Here's the drawing with two shaded views (mm, measured from the low corner). I have some questions. A direction names the side the tool comes from. Coordinates: 2 decimals unless noted, no trailing zeros. Write each loop counter-clockwise with the first axis right and the second up, starting at its lowest first coordinate (ties: lowest second). Pieces come first, ordered by that corner, then holes.
Item 1: If we section it at D-D (x = 28): Please give me the cut outline in (y, z).
Item 2: If we section it at B-B (x = 35): Please give me the cut outline in (y, z), then the cut area to 3 significant figures.
Item 3: For the marked faces 1 and 2, which set-ups out of +Z, -Z, +X, -X, +Y, -Y let a thin tool reach every point of the face, with its end or its side?
Item 4: If I drill on line 1 (X direction, y = 24.5, z = 22.5); line 2 (X direction, y = 0.8, z = 12.5); line 3 (X direction, y = 1, z = 12.5), over which ranges is the centre line in solid material (lowest first)?
Item 5: If we section it at A-A (y = 45): Please give me the cut outline in (x, z), then the cut area to 3 significant figures.
Item 6: I'm going to push flat-ended pins straight in: pin 1 Ø3.5 at (x, z) = (28, 5.5) entering from +Y; pin 2 Ø2.5 at (y, z) = (45, 12.5) entering from -X. Where does each tip first touch, or does it pass through?
Item 7: If we section it at C-C (y = 34): Please give me the cut outline in (x, z), then the cut area to 3 significant figures.
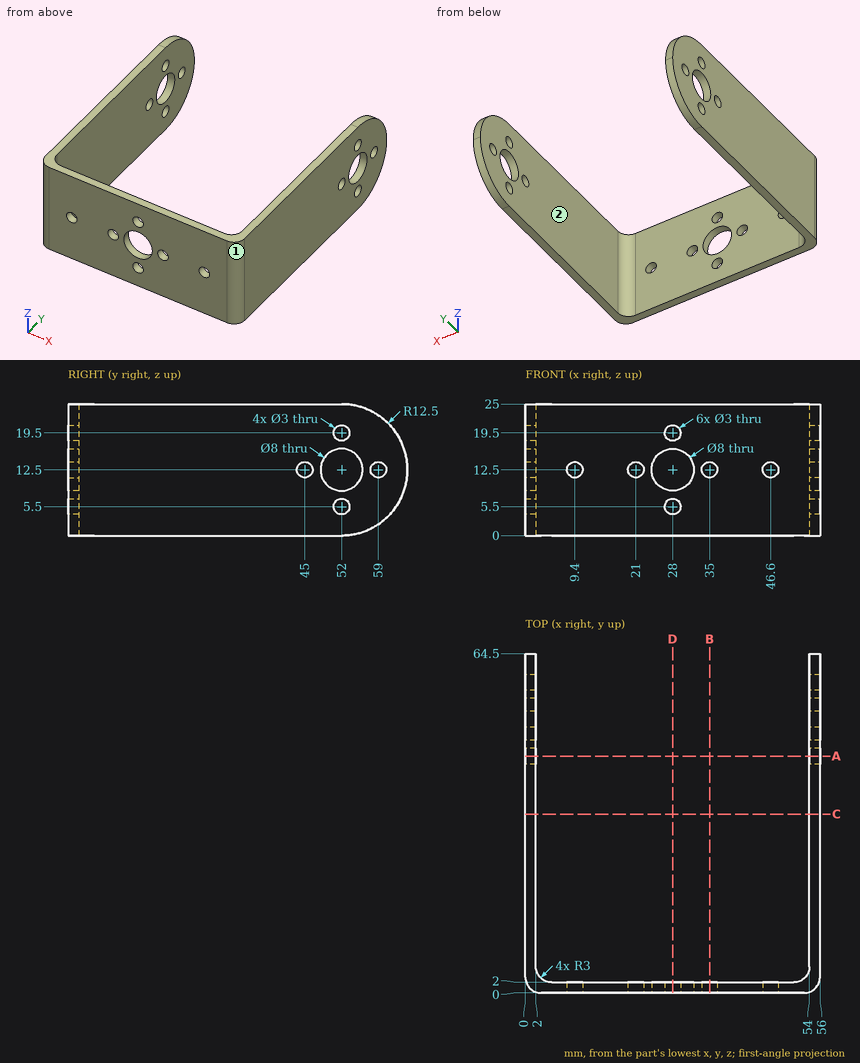
Answer list:
1. outline: (0, 0) - (2, 0) - (2, 4) - (0, 4) - close; (0, 7) - (2, 7) - (2, 8.5) - (0, 8.5) - close; (0, 16.5) - (2, 16.5) - (2, 18) - (0, 18) - close; (0, 21) - (2, 21) - (2, 25) - (0, 25) - close
2. outline: (0, 0) - (2, 0) - (2, 11) - (0, 11) - close; (0, 14) - (2, 14) - (2, 25) - (0, 25) - close
2. area: 44.0 mm2
3. face 1: +Z, -Z, +X, -Y
3. face 2: +Z, -Z, +Y
4. line 1: x = 0 to 2, 54 to 56
4. line 2: x = 0.96 to 7.9, 10.9 to 19.5, 22.5 to 24, 32 to 33.5, 36.5 to 45.1, 48.1 to 55.04
4. line 3: x = 0.76 to 7.9, 10.9 to 19.5, 22.5 to 24, 32 to 33.5, 36.5 to 45.1, 48.1 to 55.24
5. outline: (0, 0) - (2, 0) - (2, 11) - (0, 11) - close; (0, 14) - (2, 14) - (2, 25) - (0, 25) - close; (54, 0) - (56, 0) - (56, 11) - (54, 11) - close; (54, 14) - (56, 14) - (56, 25) - (54, 25) - close
5. area: 88.0 mm2
6. pin 1: stops at y = 2
6. pin 2: passes through
7. outline: (0, 0) - (2, 0) - (2, 25) - (0, 25) - close; (54, 0) - (56, 0) - (56, 25) - (54, 25) - close
7. area: 100 mm2
